Geometry check sheet. Reference: the model listing, model coordinates, mm. A direction names the side the tool comes from. Coordinates: 2 decimals unless noted, no trailing zeros.
from build123d import *

# Parameters (mm, degrees)
SKETCH8_R           = 83.841254666
BOSS_EXTRUDE1_DEPTH = 10.16
SKETCH9_R           = 117.461252673
CUT_EXTRUDE1_DEPTH  = 681.99
SKETCH10_R          = 12.7
BOSS_EXTRUDE2_DEPTH = 19.05


with BuildPart() as part:
    # Sketch7 → Revolve3 (revolve)
    with BuildSketch(Plane.XY):
        with BuildLine():
            Line((762, 83.841254666), (762, 0))
            Line((762, 0), (0, 0))
            add(Edge.make_bspline(
                [(0, 0), (0.002469036, 0.007698152), (0.00852038, 0.022545642), (0.025428785, 0.049911406), (0.065694849, 0.100096678), (0.127523873, 0.163176144), (0.212062429, 0.237272493), (0.332279694, 0.331578396), (0.47681638, 0.434147846), (0.646496772, 0.544815952), (0.841412681, 0.663024364), (1.126864222, 0.82633392), (1.572744504, 1.062892156), (2.33539055, 1.432268664), (3.710931738, 2.02979685), (6.154578127, 2.969838304), (10.668005752, 4.490267325), (18.999517068, 6.917303838), (33.385795617, 10.520869917), (58.214680344, 15.881727226), (92.501407111, 22.236378549), (134.347160824, 29.066892837), (181.232321928, 35.913847395), (228.199436648, 42.167572329), (275.229416109, 47.928683924), (322.309575865, 53.261898342), (369.432294544, 58.204857708), (416.591925172, 62.781349507), (463.784734462, 67.002125548), (511.007900045, 70.868414522), (558.259527802, 74.370378395), (605.538293137, 77.485800464), (646.930327879, 79.837294836), (682.425589554, 81.539197971), (710.863439026, 82.65535626), (729.852911101, 83.259007577), (745.309411706, 83.632760833), (754.846503834, 83.785926018), (759.61543609, 83.834878653), (762, 83.841254666)],
                knots=[0, 0, 0, 0, 0, 4.177e-05, 8.3539e-05, 0.000167079, 0.000334158, 0.000501236, 0.000668315, 0.000962463, 0.001256611, 0.001555846, 0.001855081, 0.002674694, 0.003884179, 0.005967022, 0.009661666, 0.016303633, 0.028675652, 0.051140007, 0.0868676, 0.148543873, 0.210220157, 0.271896443, 0.333572727, 0.395249011, 0.456925295, 0.518601581, 0.580277867, 0.641954151, 0.703630435, 0.765306721, 0.826983006, 0.888659291, 0.919497433, 0.950335576, 0.975167788, 0.987583894, 1, 1, 1, 1, 1], degree=4))
        make_face()
    revolve(axis=Axis((0, 0, 0), (1, 0, 0)))

    # Sketch8 → Boss-Extrude1 (add)
    with BuildSketch(Plane(origin=(762, 0, 0), x_dir=(0, 0, -1), z_dir=(1, 0, 0))):
        with Locations(Location((0, 0, 0), (0, 0, 90))):
            Circle(SKETCH8_R)
    extrude(amount=BOSS_EXTRUDE1_DEPTH)

    # Sketch9 → Cut-Extrude1 (cut)
    with BuildSketch(Plane(origin=(162.56, 0, 0), x_dir=(0, 0, -1), z_dir=(1, 0, 0))):
        Circle(SKETCH9_R)
    extrude(amount=CUT_EXTRUDE1_DEPTH, mode=Mode.SUBTRACT)

    # Sketch10 → Boss-Extrude2 (add)
    with BuildSketch(Plane(origin=(162.56, 0, 0), x_dir=(0, 0, -1), z_dir=(1, 0, 0))):
        with Locations(Location((0, 0, 0), (0, 0, 270))):
            Circle(SKETCH10_R)
    extrude(amount=BOSS_EXTRUDE2_DEPTH)


solid = part.part
(1) Access from +Z, -Z, +X, -X, +Y, -Y to the whole of each face (thin tool, end or side, straight path). Record for faces 1 (the flat face through (181.61, 0, 0)), 2 (the cylindrical face through (172, 10.1, 7.7)).
Findings:
face 1: +Z, -Z, +X, +Y, -Y
face 2: +X
(2) Gauge pin test, flat ends, axial feed: pin 1 Ø2 at (x, y) = (138.5, -10) entering from -Z; pin 2 Ø1 at (x, z) = (125.5, -7.5) entering from -Y; pin 3 Ø1.5 at (x, y) = (84, 1.5) entering from +Z. Record the tip position at first contact, or that the pin passes through.
Findings:
pin 1: stops at z = -28.17
pin 2: stops at y = -26.63
pin 3: stops at z = 20.63
(3) Scan lines: L1, parallel to Y at x = 87, z = 13.5; L2, parallel to Y at x = 66, z = 8; L3, parallel to Z at x = 90.5, y = 15.5. Record each from-to range of solid material in increasing order.
Findings:
L1: y = -16.19 to 16.19
L2: y = -15.24 to 15.24
L3: z = -15.18 to 15.18
